The listing builds one solid part. Answer for the finished solid, in the listing's coordinates (mm). A direction names the side the tool comes from. Round coordinates to 2 decimals unless told otherwise and drop trailing zeros. Order: outer loops, then holes, each group sorted by start corner. A loop starts at its lowest first (then second) coordinate and runs counter-clockwise, first axis right, second up. Notation, with made-up numbers: (-10.5, -17.5) - (43.5, -17.5) arc R17 cw to (43.5, 10.5) - close; hole circle Ø6 at (2, 50.25). An arc over 180 degrees is marked (long way). Use CSV: the item, a comma, the result in double quotes. Start each with the question number.
Item 1: For faces 1 (the flat face through (0, 0, 10)), 2 (the flat face through (-1, 1, 52)), 3 (the flat face through (-5, -8, 2)), 4 (the flat face through (10, 0, 2)), 5 (the flat face through (-1, 8, 27)), determine the directions among +Z, -Z, +X, -X, +Y, -Y from which every point of the face is accessible in a straight line to the end or side of a thin tool.
Item 2: Flat-ended cylindrical pins translate along their axes: P1, Ø8, axis at y = 7.5, z = 9.5, coming from the +X side; P2, Ø4, axis at x = 8, y = 9, coming from the +Z side; P3, Ø6, axis at y = -5.5, z = 20.5, coming from the -X side. Find the tip coordinate at first contact, or state that the pin passes through.
Item 3: Determine the mould class of faces 6 (the flat face through (1, 8, 27)), 7 (the flat face through (-6.387, 4.842, 26.65)), 8 (the flat face through (7.39, 3.11, 26.65)) for opening direction Y: +Y half, -Y half, draft (parallel to the pull), parting line (faces both ways), or undercut.
Item 4: Find section A-A, the plane z = 32.5. Give the vertices of the cut face in (x, y), plus the area to 3 significant figures.
Item 5: Straight lines are drawn through the part: line 1 along Z through (x, y) = (-2.75, -0.5); line 2 along Z through (x, y) = (-1.5, 6.5); line 3 along Y through (x, z) = (-3.25, 47). For each, find the intervals that lie inside material, in ascending order. Write a range as [from, to].
```python
from build123d import *
from build123d.topology import SkipClean

# Parameters (mm, degrees)
SKETCH1_R           = 15
BOSS_EXTRUDE1_DEPTH = 2
BOSS_EXTRUDE2_DEPTH = 50
CIRPATTERN1_COUNT   = 3
CIRPATTERN1_ANGLE   = 120
CUT_EXTRUDE1_DEPTH  = 10
FILLET2_R           = 1
FILLET3_R           = 1


with BuildPart() as part:
    # Sketch1 → Boss-Extrude1 (new body)
    with BuildSketch(Plane.XY):
        Circle(SKETCH1_R)
    extrude(amount=BOSS_EXTRUDE1_DEPTH)

    # Sketch2 → Boss-Extrude2 (add)
    with SkipClean():  # the faces are left unmerged after this step: merging them gives an invalid solid
        with BuildSketch(Plane.XY.offset(2)):
            with BuildLine():
                Line((-1, -14.966629547), (-1, 14.966629547))
                ThreePointArc((-1, 14.966629547), (0, 15), (1, 14.966629547))
                Line((1, 14.966629547), (1, -14.966629547))
                ThreePointArc((1, -14.966629547), (0, -15), (-1, -14.966629547))
            make_face()
        boss_extrude2 = extrude(amount=BOSS_EXTRUDE2_DEPTH)

    # CirPattern1: Boss-Extrude2 ×3 about axis
    with SkipClean():  # the faces are left unmerged after this step: merging them gives an invalid solid
        cirpattern1_axis = Axis((0, 0, 0), (0, 0, 1))
        for i in range(1, CIRPATTERN1_COUNT):
            add(boss_extrude2.rotate(cirpattern1_axis, i * CIRPATTERN1_ANGLE / (CIRPATTERN1_COUNT - 1)))

    # Sketch3 → Cut-Extrude1 (cut)
    with SkipClean():  # the faces are left unmerged after this step: merging them gives an invalid solid
        with BuildSketch(Plane(origin=(0, 0, 0), x_dir=(-1, 0, 0), z_dir=(0, 0, -1))):
            with BuildLine():
                Line((-2.598076211, 1.5), (2.598076211, 1.5))
                ThreePointArc((2.598076211, 1.5), (0, -3), (-2.598076211, 1.5))
            make_face()
        extrude(amount=-CUT_EXTRUDE1_DEPTH, mode=Mode.SUBTRACT)

    # Fillet2
    # the kernel refuses this fillet: 1 mm, written as the material it takes off along each edge
    with BuildSketch(Plane(origin=(12.461481397, 8.349340177, 2), x_dir=(0.5286054177499072, -0.8488676647896573, 0), z_dir=(0, 0, 1)), Plane(origin=(-12.461481397, -8.349340177, 2), x_dir=(-0.5286054177499102, 0.8488676647896556, 0), z_dir=(0, 0, 1)), Plane(origin=(-13.461481397, 6.61728937, 2), x_dir=(0.4708382532840629, 0.882219552744334, 0), z_dir=(0, 0, 1)), Plane(origin=(13.461481397, -6.61728937, 2), x_dir=(-0.47083825328406437, -0.8822195527443331, 0), z_dir=(0, 0, 1)), Plane(origin=(-1, 14.966629547, 2), x_dir=(0.9994436710339702, 0.03335188795467453, 0), z_dir=(0, 0, 1)), Plane(origin=(1, -14.966629547, 2), x_dir=(-0.9994436710339702, -0.03335188795467453, 0), z_dir=(0, 0, 1))) as fillet2_piece_1:
        with BuildLine():
            CenterArc((0.967204751, -0.999443671), FILLET2_R, 88.088723135, 90)
            Line((-0.03223892, -0.966091783), (0, 0))
            ThreePointArc((0, 0), (0.500278319, 0.008344934), (1.000556639, 0))
        make_face()
    extrude(amount=52.501391597, mode=Mode.SUBTRACT)
    with BuildSketch(Plane(origin=(-12.461481397, 8.349340177, 2), x_dir=(-0.5286054177498939, -0.8488676647896658, 0), z_dir=(0, 0, 1)), Plane(origin=(12.461481397, -8.349340177, 2), x_dir=(0.52860541774991, 0.8488676647896555, 0), z_dir=(0, 0, 1)), Plane(origin=(13.461481397, 6.61728937, 2), x_dir=(-0.4708382532840634, 0.8822195527443337, 0), z_dir=(0, 0, 1)), Plane(origin=(-13.461481397, -6.61728937, 2), x_dir=(0.470838253284063, -0.8822195527443338, 0), z_dir=(0, 0, 1)), Plane(origin=(1, 14.966629547, 2), x_dir=(-0.9994436710339702, 0.03335188795467452, 0), z_dir=(0, 0, 1)), Plane(origin=(-1, -14.966629547, 2), x_dir=(0.9994436710339702, -0.03335188795467453, 0), z_dir=(0, 0, 1))) as fillet2_piece_2:
        with BuildLine():
            CenterArc((0.967204751, 0.999443671), FILLET2_R, 181.911276865, 90)
            Line((-0.03223892, 0.966091783), (0, 0))
            ThreePointArc((0, 0), (0.500278319, -0.008344934), (1.000556639, 0))
        make_face()
    extrude(amount=52.501391597, mode=Mode.SUBTRACT)

    # Fillet3
    fillet3_edges = [part.edges().sort_by_distance(p)[0] for p in [
        (-15, 0, 0),
    ]]
    fillet(fillet3_edges, radius=FILLET3_R)


solid = part.part
```
Worked out:
1,face 1,"-Z"
1,face 2,"+Z, +X, -X, +Y, -Y"
1,face 3,"+Z, -Y"
1,face 4,"+Z, +X"
1,face 5,"+Z, +Y"
2,P1,"stops at x = 13.12"
2,P2,"stops at z = 2"
2,P3,"stops at x = -13.12"
3,face 6,"draft"
3,face 7,"+Y half"
3,face 8,"undercut"
4,outline,"(-12.62, -6.13) arc R1 ccw to (-11.62, -7.87) - (-1, -1.73) - (-1, -14) arc R1 ccw to (1, -14) - (1, -1.73) - (11.62, -7.87) arc R1 ccw to (12.62, -6.13) - (2, 0) - (12.62, 6.13) arc R1 ccw to (11.62, 7.87) - (1, 1.73) - (1, 14) arc R1 ccw to (-1, 14) - (-1, 1.73) - (-11.62, 7.87) arc R1 ccw to (-12.62, 6.13) - (-2, 0) - close"
4,area,"167 mm²"
5,line 1,"z = [10, 52]"
5,line 2,"z = [0, 2]"
5,line 3,"y = [-3.03, -0.72], [0.72, 3.03]"
